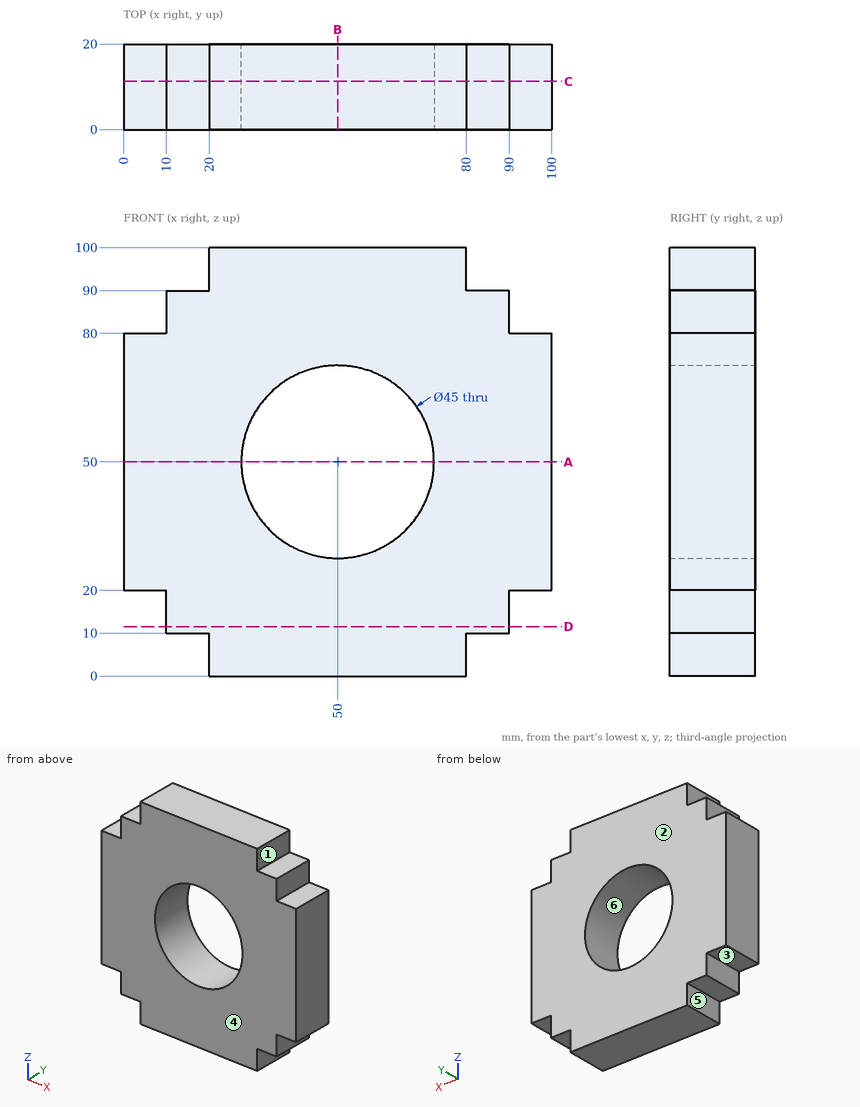
Drawing for the job (mm, zero at the part's lowest x, y, z). A direction names the side the tool comes from. Round coordinates to 2 decimals unless told otherwise and drop trailing zeros. Write each loop counter-clockwise with the first axis right and the second up, starting at its lowest first coordinate (ties: lowest second). Pieces come first, ordered by that corner, then holes. Notation, with made-up numbers: M 79.5,88 L 115.5,88 A21 ccw 115.5,125 Z; hole C 37,15.5 d10. An arc over 180 degrees is marked long. Answer as a JSON object with one key per item and string values. Group by question number.
(1) Cut at D-D (z = 11.5). Give the cut face in (x, y).
(2) Which spindle directions (+Z, -Z, +X, -X, +Y, -Y) get a long thin tool onto all of the face, cutting with end or side? Do the marked faces 1, 2 and 3. Say none if no direction does.
(3) Drill centre lines: L1, parallel to Z at x = 50, y = 13.75; L2, parallel to X at y = 6.5, z = 13; L3, parallel to Z at x = 7.5, y = 18.5. Where is each one in solid material? Low to high.
(4) Cut at B-B (x = 50). Give the cut face in (y, z), and give its area (3 significant figures).
(5) Cut at A-A (z = 50). Give the cut face in (x, y), and give its area (3 significant figures).
(6) Flat gauge pins, fed straight in: pin 1 (3 mm diameter, centred on x = 96, y = 5.5, fed in from -Z); pin 2 (1 mm diameter, centred on y = 14.5, z = 89.5, fed in from +X); pin 3 (3 mm diameter, centred on x = 83.5, y = 8, fed in from -Z); pin 4 (10 mm diameter, centred on y = 8, z = 21.5, fed in from -X). Where does each tip first touch, or does it go through?
(7) Mould opens along X. For the marked faces 4, 5 and 6 say: pulls with the +X half, pulls with the -X half, needs draft (parallel to the pull), parting line crosses it, or undercut.
(8) Cut at C-C (y = 11.25). Give the cut face in (x, z).
Responses:
{
 "1": {"outline": "M 10,0 L 90,0 L 90,20 L 10,20 Z"},
 "2": {"face 1": "+Z, +X, +Y, -Y", "face 2": "+Z, -Z, +X, -X, +Y", "face 3": "-Z, -X, +Y, -Y"},
 "3": {"L1": "z = 0 to 27.5, 72.5 to 100", "L2": "x = 10 to 90", "L3": "z = 20 to 80"},
 "4": {"outline": "M 0,0 L 20,0 L 20,27.5 L 0,27.5 Z; M 0,72.5 L 20,72.5 L 20,100 L 0,100 Z", "area": "1,100 mm2"},
 "5": {"outline": "M 0,0 L 27.5,0 L 27.5,20 L 0,20 Z; M 72.5,0 L 100,0 L 100,20 L 72.5,20 Z", "area": "1,100 mm2"},
 "6": {"pin 1": "stops at z = 20", "pin 2": "stops at x = 90", "pin 3": "stops at z = 10", "pin 4": "stops at x = 0"},
 "7": {"face 4": "needs draft", "face 5": "pulls with the -X half", "face 6": "undercut"},
 "8": {"outline": "M 0,20 L 10,20 L 10,10 L 20,10 L 20,0 L 80,0 L 80,10 L 90,10 L 90,20 L 100,20 L 100,80 L 90,80 L 90,90 L 80,90 L 80,100 L 20,100 L 20,90 L 10,90 L 10,80 L 0,80 Z; hole C 50,50 d45"}
}
